Autodesk Inventor part; units mm, degrees
ref_plane "YZ Plane" through (0, 0, 0) normal (1, 0, 0) x (0, 1, 0)
ref_plane "XZ Plane" through (0, 0, 0) normal (0, 1, 0) x (-1, 0, 0)
ref_plane "XY Plane" through (0, 0, 0) normal (0, 0, 1) x (1, 0, 0)
sketch "Sketch3" plane through (0, 0, 0) normal (0, 0, 1) x (1, 0, 0)
  line L0 (0, 0) -> (266.7, 0)
  line L1 (266.7, 0) -> (266.7, -152.4)
  line L2 (266.7, -152.4) -> (0, -152.4)
  line L3 (0, -152.4) -> (0, 0)
  dimension "d8" = 266.7
  dimension "d9" = 152.4
extrude "Extrusion3" add sketch "Sketch3" along normal blind 5.08
sketch "Sketch4" plane through (0, 0, 5.08) normal (0, 0, 1) x (1, 0, 0)
  line L0 (0, -152.4) -> (266.7, -152.4)
  line L1 (266.7, 0) -> (0, 0)
  line L2 (133.35, 0) -> (133.35, -152.4)
  line L3 (266.7, -152.4) -> (266.7, 0)
  circle A0 centre (126.492, -28.2016) radius 1.651
  circle A1 centre (140.208, -28.2016) radius 1.651
  circle A2 centre (191.77, -28.2016) radius 1.651
  circle A3 centre (74.93, -28.2016) radius 1.651
  circle A4 centre (205.486, -28.2016) radius 1.651
  circle A5 centre (61.214, -28.2016) radius 1.651
  circle A6 centre (257.048, -28.2016) radius 1.651
  circle A7 centre (9.652, -28.2016) radius 1.651
  circle A8 centre (140.208, -63.7616) radius 1.651
  circle A9 centre (126.492, -63.7616) radius 1.651
  circle A10 centre (191.77, -63.7616) radius 1.651
  circle A11 centre (74.93, -63.7616) radius 1.651
  circle A12 centre (205.486, -63.7616) radius 1.651
  circle A13 centre (61.214, -63.7616) radius 1.651
  circle A14 centre (257.048, -63.7616) radius 1.651
  circle A15 centre (9.652, -63.7616) radius 1.651
  circle A16 centre (153.162, -45.9816) radius 2.413
  circle A17 centre (113.538, -45.9816) radius 2.413
  circle A18 centre (178.816, -45.9816) radius 2.413
  circle A19 centre (87.884, -45.9816) radius 2.413
  circle A20 centre (218.44, -45.9816) radius 2.413
  circle A21 centre (48.26, -45.9816) radius 2.413
  circle A22 centre (244.094, -45.9816) radius 2.413
  circle A23 centre (22.606, -45.9816) radius 2.413
extrude "Extrusion5" cut sketch "Sketch4" against normal blind 25.4 contours A0 | A1 | A2 | A3 | A4 | A5 | A6 | A7 | A8 | A9 | A10 | A11 | A12 | A13 | A14 | A15 | A16 | A17 | A18 | A19 | A20 | A21 | A22 | A23
sketch "Sketch6" plane through (0, 0, 5.08) normal (0, 0, 1) x (1, 0, 0)
  circle A0 centre (22.606, -45.9816) radius 2.413
  circle A1 centre (48.26, -45.9816) radius 2.413
  circle A2 centre (87.884, -45.9816) radius 2.413
  circle A3 centre (113.538, -45.9816) radius 2.413
  line L0 (266.7, 0) -> (0, 0)
  line L1 (0, 0) -> (266.7, 0)
  line L2 (133.35, 0) -> (133.35, -152.4)
  line L3 (0, -152.4) -> (266.7, -152.4)
  circle A4 centre (35.433, -134.8816) radius 6.35
  circle A5 centre (100.711, -134.8816) radius 6.35
  circle A6 centre (231.267, -134.8816) radius 6.35
  circle A7 centre (165.989, -134.8816) radius 6.35
  dimension "d99" = 12.7
  dimension "d100" = 12.7
extrude "Extrusion6" cut sketch "Sketch6" against normal blind 25.4 contours A4 | A5 | A6 | A7
sketch "Sketch7" plane through (0, 0, 5.08) normal (0, 0, 1) x (1, 0, 0)
  point P0 (0, 0)
sketch "Sketch8" plane through (0, 0, 5.08) normal (0, 0, 1) x (1, 0, 0)
  line L0 (266.7, 0) -> (0, 0)
  line L1 (0, -152.4) -> (266.7, -152.4)
  circle A0 centre (165.989, -134.8816) radius 6.35
  circle A1 centre (231.267, -134.8816) radius 6.35
sketch "Sketch9" plane through (0, 0, 5.08) normal (0, 0, 1) x (1, 0, 0)
  line L0 (266.7, 0) -> (0, 0)
  line L1 (133.35, 0) -> (133.35, -152.4)
  line L2 (0, -152.4) -> (266.7, -152.4)
properties part number "Back wall"
The listing builds one solid part. Answer for the finished solid, in the listing's coordinates (mm). Coordinates: 2 decimals unless noted, no trailing zeros. Put each result on its own line as item: value. Start each with the question number.
1. A cutting plane is placed at A-A on z = 1. Count the separate pieces of the cut face and the enclosed holes in it, then the cut area to 3 significant figures.
2. Consider line 1 (X direction, y = -130.5, z = 2.9); line 2 (Y direction, x = 24, z = 0.35); line 3 (Y direction, x = 162, z = 2.65). Determine where each line is inside the solid, lowest interval first. Write a range as from..to.
3. For a pull along Y with two mould halves and no side action, classify faces 1 (the cylindrical face through (246.396, -45.257, 2.576)), 2 (the cylindrical face through (181.12, -45.26, 2.58)), 3 (the flat face through (135, -152.4, 3)), 4 (the flat face through (131, -75, 0)) as pulls with the +Y half, pulls with the -Y half, needs draft (parallel to the pull), parting line crosses it, or undercut.
4. A flat-ended cylindrical pin translates along its axis: P1, Ø2, axis at x = 61.21, y = -63.76, coming from the +Z side. Find the tip coordinate at first contact, or state that the pin passes through.
Resolved:
1. separate pieces: 1
1. enclosed holes: 28
1. area: 39,900 mm2
2. line 1: x = 0..30.84, 40.03..96.11, 105.31..161.39, 170.59..226.67, 235.86..266.7
2. line 2: y = -152.4..-47.95, -44.01..0
2. line 3: y = -152.4..-139.82, -129.94..0
3. face 1: undercut
3. face 2: undercut
3. face 3: pulls with the -Y half
3. face 4: needs draft
4. P1: passes through
